from build123d import *

# Parameters (mm, degrees)
BOSS_EXTRUDE1_DEPTH = 203.2
SKETCH2_OUTSIDE_W   = 72.704
SKETCH2_OUTSIDE_H   = 68.774
SKETCH2_OUTSIDE_R   = 7.9375
CUT_EXTRUDE1_DEPTH  = 25.4
CUT_EXTRUDE3_START  = -177.8
SKETCH2_2_OUTSIDE_W = 72.704
SKETCH2_2_OUTSIDE_H = 68.774
SKETCH2_2_OUTSIDE_R = 7.9375
CUT_EXTRUDE3_DEPTH  = 25.4


with BuildPart() as part:
    # Sketch1 → Boss-Extrude1 (new body)
    with BuildSketch(Plane(origin=(0, 0, 0), x_dir=(0, 0, -1), z_dir=(1, 0, 0))):
        Polygon((14.664696837, 0), (7.332348419, 12.7), (-7.332348419, 12.7), (-14.664696837, 0), (-7.332348419, -12.7), (7.332348419, -12.7), align=None)
    extrude(amount=BOSS_EXTRUDE1_DEPTH)

    # Sketch2 outside → Cut-Extrude1 (cut)
    with BuildSketch(Plane(origin=(203.2, 0, 0), x_dir=(0, 0, -1), z_dir=(1, 0, 0))):
        Rectangle(SKETCH2_OUTSIDE_W, SKETCH2_OUTSIDE_H)
        Circle(SKETCH2_OUTSIDE_R, mode=Mode.SUBTRACT)
    extrude(amount=-CUT_EXTRUDE1_DEPTH, mode=Mode.SUBTRACT)

    # Sketch2<2> outside → Cut-Extrude3 (cut)
    with BuildSketch(Plane(origin=(203.2, 0, 0), x_dir=(0, 0, -1), z_dir=(1, 0, 0)).offset(CUT_EXTRUDE3_START)):
        Rectangle(SKETCH2_2_OUTSIDE_W, SKETCH2_2_OUTSIDE_H)
        Circle(SKETCH2_2_OUTSIDE_R, mode=Mode.SUBTRACT)
    extrude(amount=-CUT_EXTRUDE3_DEPTH, mode=Mode.SUBTRACT)


solid = part.part
Work out the finished part from the listing and answer in its coordinate system (mm). A direction names the side the tool comes from. Give positions to 0.01 mm unless a question says otherwise; leave off trailing zeros. Write each loop counter-clockwise with the first axis right and the second up, starting at its lowest first coordinate (ties: lowest second). Pieces come first, ordered by that corner, then holes.
Q1. The part is cut by section A-A on z = 0. Give the vertices of the cut face in (x, y).
Answer:
outline: (0, -7.94) - (25.4, -7.94) - (25.4, -12.7) - (177.8, -12.7) - (177.8, -7.94) - (203.2, -7.94) - (203.2, 7.94) - (177.8, 7.94) - (177.8, 12.7) - (25.4, 12.7) - (25.4, 7.94) - (0, 7.94) - close
Q2. The part is cut by section C-C on y = 2.75. Give the vertices of the cut face in (x, z), and give its area (3 significant figures).
Answer:
outline: (0, -7.45) - (25.4, -7.45) - (25.4, -13.08) - (177.8, -13.08) - (177.8, -7.45) - (203.2, -7.45) - (203.2, 7.45) - (177.8, 7.45) - (177.8, 13.08) - (25.4, 13.08) - (25.4, 7.45) - (0, 7.45) - close
area: 4,740 mm2
Q3. The part is cut by section B-B on x = 87.5. Give the vertices of the cut face in (y, z).
Answer:
outline: (-12.7, -7.33) - (0, -14.66) - (12.7, -7.33) - (12.7, 7.33) - (0, 14.66) - (-12.7, 7.33) - close
Q4. A tool of negligible diameter and unlimited length cuts with its end or side. For faces 1 (the face through (25.4, 6, -6)), 2 (the face through (203.2, 0, 0)), 3 (the face through (177.8, 6, -6)), from which of +Z, -Z, +X, -X, +Y, -Y can it reach the whole face along a straight path? Write none if from no direction.
Answer:
face 1: -X
face 2: +Z, -Z, +X, +Y, -Y
face 3: +X
Q5. The part is cut by section D-D on y = 10.25. Give the vertices of the cut face in (x, z).
Answer:
outline: (25.4, -8.75) - (177.8, -8.75) - (177.8, 8.75) - (25.4, 8.75) - close
Q6. Straight lines are drawn through the part: L1, parallel to X at y = 8.5, z = -8; L2, parallel to Y at x = 81, z = -11; L3, parallel to Z at x = 47, y = 9. For each, find the intervals that lie inside material, in ascending order.
Answer:
L1: x = 25.4 to 177.8
L2: y = -6.35 to 6.35
L3: z = -9.47 to 9.47
Q7. Given pin 1 (1 mm diameter, centred on x = 148, y = 3.5, fed in from -Z); pin 2 (1.5 mm diameter, centred on x = 21, y = 3, fed in from +Z); pin 3 (1.5 mm diameter, centred on x = 118.5, y = -0.5, fed in from +Z), each flat-ended and moving along its own axis, determine where each tip first touches the part or whether it passes through.
Answer:
pin 1: stops at z = -12.93
pin 2: stops at z = 7.61
pin 3: stops at z = 14.66
